Autodesk Inventor part; units mm, degrees
ref_plane "YZ Plane" through (0, 0, 0) normal (1, 0, 0) x (0, 1, 0)
ref_plane "XZ Plane" through (0, 0, 0) normal (0, 1, 0) x (-1, 0, 0)
ref_plane "XY Plane" through (0, 0, 0) normal (0, 0, 1) x (1, 0, 0)
sketch "Sketch1" plane through (0, 0, 0) normal (0, 1, 0) x (-1, 0, 0)
  line L0 (25.7143, 25.1429) -> (-22.2857, 25.1429)
  line L1 (-22.2857, 25.1429) -> (-22.2857, -14.8571)
  line L2 (-22.2857, -14.8571) -> (25.7143, -14.8571)
  line L3 (25.7143, -14.8571) -> (25.7143, 25.1429)
  circle A0 centre (18.7143, 15.1429) radius 2.75
  circle A1 centre (18.7143, -4.8571) radius 2.75
  circle A2 centre (4.7143, -4.8571) radius 2.75
  circle A3 centre (4.7143, 15.1429) radius 2.75
  circle A4 centre (-12.2857, 15.1429) radius 2.75
  circle A5 centre (-12.2857, -4.8571) radius 2.75
  point P0 (0, 0)
  dimension "d0" = 48
  dimension "d1" = 40
  dimension "d2" = 5.5
  dimension "d3" = 5.5
  dimension "d4" = 5.5
  dimension "d5" = 5.5
  dimension "d6" = 5.5
  dimension "d7" = 5.5
  dimension "d8" = 7
  dimension "d9" = 14
  dimension "d10" = 17
  dimension "d12" = 20
  dimension "d13" = 10
  dimension "d24" = 10
extrude "Extrusion1" add sketch "Sketch1" along normal blind 4
sketch "Sketch3" plane through (0, 4, 0) normal (0, 1, 0) x (1, 0, 0)
  line L0 (22.2857, -25.1429) -> (22.2857, 14.8571)
  line L1 (-25.7143, -25.1429) -> (22.2857, -25.1429)
  line L2 (22.2857, 14.8571) -> (2.2857, 14.8571)
  line L3 (2.2857, 14.8571) -> (2.2857, -25.1429)
  line L4 (2.2857, -25.1429) -> (22.2857, -25.1429)
  line L5 (22.2857, -25.1429) -> (22.2857, 14.8571)
  point P0 (0, 0)
  dimension "d17" = 20
extrude "Extrusion2" add sketch "Sketch3" along normal blind 4
sketch "Sketch4" plane through (12.2857, 4, 15.1429) normal (0, -1, 0) x (1, 0, 0)
  circle A0 centre (0, 0) radius 2.75
  circle A1 centre (0, -20) radius 2.75
  circle A2 centre (0, -20) radius 2.75
  point P0 (-12.2857, -15.1429)
extrude "Extrusion3" cut sketch "Sketch4" against normal blind 4
fillet "Fillet2" radius 2 10 edges at (-1.7143, 0, -14.8571) (22.2857, 4, -14.8571) (22.2857, 0, 5.1429) (-1.7143, 0, 25.1429) (-25.7143, 0, 5.1429) (-25.7143, 4, 5.1429) (-11.7143, 4, 25.1429) (-11.7143, 4, -14.8571) (22.2857, 8, 5.1429) (22.2857, 4, 25.1429)
fillet "Fillet3" radius 1.5 4 edges at (2.2857, 3.0003, 25.1429) (2.2857, 6, 25.1429) (2.2857, 6, -14.8571) (2.2857, 3.0003, -14.8571)
properties part number "syringepumpplate_bottom"
Could you check a few things on this model? Use its own coordinates, in mm. A direction names the side the tool comes from. Round coordinates to 2 decimals unless told otherwise and drop trailing zeros. Write each loop counter-clockwise with the first axis right and the second up, starting at its lowest first coordinate (ties: lowest second). Pieces come first, ordered by that corner, then holes. Notation, with made-up numbers: (42, 89.25) - (66, 89.25) arc R16 cw to (66, 116.25) - close; hole circle Ø1 at (32, 42). An arc over 180 degrees is marked (long way). Put each result on its own line as item: value. Start each with the question number.
(1) I need wall thicknesses on probe 1 along Z at (x, y) = (-20.5, 1.5); probe 2 along Z at (x, y) = (-20.5, 1); probe 3 along Y at (x, z) = (-4, 21.5). Which ranges of each line are inside material? Lowest first, please.
(2) I want a section at C-C, the plane y = 1.25. Please give me the cut outline in (x, z).
(3) For faces 1 (the flat face through (-11, 4, 5)), 2 (the cylindrical face through (-3.036, 0.601, -14.287)), 3 (the flat face through (11, 5, -14.857)), 4 (the cylindrical face through (-11.171, 3.43, -14.256)), 5 (the cylindrical face through (-10.76, 3.43, 24.54)), which set-ups out of +Z, -Z, +X, -X, +Y, -Y let a thin tool reach every point of the face, with its end or its side?
(4) Thinking about a two-plate mould opening in X: for faces 6 (the flat face through (13, 5, 25.143)), 7 (the cylindrical face through (2.74, 5.62, 24.72)), 8 (the cylindrical face through (-4.118, 1.972, 17.828)), which applies, released by +X, released by -X, zero draft, split by the parting line, or undercut?
(5) Will these pins go through, and if not, where does the flat tip stop? pin 1 (4.5 mm diameter, centred on x = -18.71, z = -4.86, fed in from -Y); pin 2 (1.2 mm diameter, centred on y = 6, z = -2.5, fed in from -X); pin 3 (21 mm diameter, centred on x = -10.5, z = 4.5, fed in from +Y).
(6) I want a section at A-A, the plane z = -5.5. Give the number of separate pieces and of enclosed holes in the cut face, plus the area to 3 significant figures.
Here are the results:
1. probe 1: z = -14.79 to -6.95, -2.77 to 13.05, 17.23 to 25.08
1. probe 2: z = -14.59 to -6.95, -2.77 to 13.05, 17.23 to 24.88
1. probe 3: y = 0 to 4
2. outline: (-25.57, -14.71) - (20.29, -14.71) arc R1.85 ccw to (22.14, -12.86) - (22.14, 23.14) arc R1.85 ccw to (20.29, 25) - (-25.57, 25) - close; hole circle Ø5.5 at (-18.71, -4.86); hole circle Ø5.5 at (-18.71, 15.14); hole circle Ø5.5 at (-4.71, -4.86); hole circle Ø5.5 at (-4.71, 15.14); hole circle Ø5.5 at (12.29, -4.86); hole circle Ø5.5 at (12.29, 15.14)
3. face 1: +Z, -Z, -X, +Y
3. face 2: -Z, +X, -X, -Y
3. face 3: -Z, +X, -X, +Y, -Y
3. face 4: -Z, -X, +Y
3. face 5: +Z, -X, +Y
4. face 6: zero draft
4. face 7: released by -X
4. face 8: undercut
5. pin 1: passes through
5. pin 2: stops at x = 2.29
5. pin 3: stops at y = 4
6. separate pieces: 4
6. enclosed holes: 0
6. area: 183 mm^2
